Design review of the part built by this model. Coordinates are the model's own, in mm. A direction names the side the tool comes from. Round coordinates to 2 decimals unless told otherwise and drop trailing zeros. Loops run counter-clockwise (first coordinate to the right, second up) from the corner with the lowest first, then second, coordinate; pieces in that order, holes last. Notation, with made-up numbers: (29.5, 34.5) -> (68.5, 34.5) arc R24 cw to (68.5, 55.5) -> close; hole circle Ø4 at (-20, 63). An arc over 180 degrees is marked (long way). Answer as CSV lines item,"result". Start each with the question number.
(1) Take a section at B-B, the plane z = 10. Write out the cut boundary in (x, y), and give its area (3 significant figures).
(2) For P1, Ø4, axis at x = 43, y = 15.5, coming from the -Z side; P2, Ø12, axis at y = 11.5, z = 23.5, coming from the -X side; P3, Ø5, axis at y = 8.5, z = 10.5, coming from the -X side, all flat-tipped, find the tip position at first contact; note any pin that passes through.
(3) Take a section at D-D, the plane z = -10. Write out the cut boundary in (x, y).
(4) Take a section at C-C, the plane y = 28. Write out the cut boundary in (x, z).
(5) Take a section at A-A, the plane x = 35. Write out the cut boundary in (y, z).
(6) Machinability: for faces 1 (the face through (-39.643, 17.283, -13.252)), 2 (the face through (-38, 34, 11)), which of the approach directions +Z, -Z, +X, -X, +Y, -Y give a long, thin tool a straight path to every point of the face, cutting with its end or side? Answer none if there is none.
(7) To check wall thickness, follow line 1 (X direction, y = 13, z = 10); line 2 (Z direction, x = 35, y = 12); line 3 (X direction, y = 24.5, z = -10). State the ranges of each line that lie inside material, in increasing order. Write a range as from..to.
(8) Draft analysis for pull direction X (two halves, no side actions). For faces 3 (the face through (-11.581, 1.875, -3.021)), 4 (the face through (30, 17, 40)), 5 (the face through (-40, 16, 12)), state which applies: +X half, -X half, draft (parallel to the pull), parting line (faces both ways), or undercut.
from build123d import *
from OCP.BRepFilletAPI import BRepFilletAPI_MakeChamfer

# Parameters (mm, degrees)
BOSS_EXTRUDE1_DEPTH     = 35
CUT_EXTRUDE3_DEPTH      = 84.964278119
CUT_EXTRUDE3_DEPTH_BACK = 84.964278119
SKETCH2_R               = 12.5
SKETCH2_R_2             = 15
CHAMFER1_SIZE           = 3
CHAMFER2_SIZE           = 2
CHAMFER3_SIZE           = 5
CHAMFER3_SIZE2          = 2.886751346
FILLET1_R               = 5


with BuildPart() as part:
    # Sketch1 → Boss-Extrude1 (new body)
    with BuildSketch(Plane(origin=(0, 0, 0), x_dir=(1, 0, 0), z_dir=(0, 1, 0))):
        with BuildLine():
            Line((-40, -16.905989232), (0, -40))
            Line((0, -40), (65, -40))
            Line((65, -40), (65, 20))
            Line((65, 20), (-4.844355629, 20))
            ThreePointArc((-4.844355629, 20), (-38.631222116, 27.900831925), (-40, -6.770509831))
            Line((-40, -6.770509831), (-40, -16.905989232))
        make_face()
    extrude(amount=BOSS_EXTRUDE1_DEPTH)

    # Sketch2 → Cut-Extrude3 (cut, two sides: drawn at the far end of the back side and taken through both)
    with BuildSketch(Plane(origin=(0, 0, 0), x_dir=(1, 0, 0), z_dir=(0, 1, 0)).offset(-CUT_EXTRUDE3_DEPTH_BACK)):
        with Locations(Location((35, -10, 0), (0, 0, 270))):
            Circle(SKETCH2_R)
        with Locations(Location((-25, 10, 0), (0, 0, 270))):
            Circle(SKETCH2_R_2)
    extrude(amount=CUT_EXTRUDE3_DEPTH + CUT_EXTRUDE3_DEPTH_BACK, mode=Mode.SUBTRACT)

    # Chamfer1
    chamfer1_edges = [part.edges().sort_by_distance(p)[0] for p in [
        (-20, 35, 28.452994616),
        (-40, 35, 11.838249532),
        (-38.631222116, 35, -27.900831925),
    ]]
    chamfer(chamfer1_edges, length=CHAMFER1_SIZE)

    # Chamfer2
    chamfer2_edges = [part.edges().sort_by_distance(p)[0] for p in [
        (-25, 0, -25),
        (-25, 35, -25),
    ]]
    chamfer(chamfer2_edges, length=CHAMFER2_SIZE)

    # Chamfer3: one chamfer whose edges measure the first distance from different faces: ONE call of the kernel's chamfer builder (chamfer() names one face for all edges)
    chamfer3_edges_1 = [part.edges().sort_by_distance(p)[0] for p in [
        (35, 0, -2.5),
    ]]
    chamfer3_side_1 = [part.faces().sort_by_distance(p)[0] for p in [
        (35, 17.5, -2.5),
    ]]
    chamfer3_edges_2 = [part.edges().sort_by_distance(p)[0] for p in [
        (35, 35, -2.5),
    ]]
    chamfer3_side_2 = [part.faces().sort_by_distance(p)[0] for p in [
        (20.131502665, 35, 9.160583392),
    ]]
    chamfer3 = BRepFilletAPI_MakeChamfer(part.part.solid().wrapped)
    for e in chamfer3_edges_1:
        chamfer3.Add(CHAMFER3_SIZE, CHAMFER3_SIZE2, e.wrapped, chamfer3_side_1[0].wrapped)  # the first distance lies on this face
    for e in chamfer3_edges_2:
        chamfer3.Add(CHAMFER3_SIZE, CHAMFER3_SIZE2, e.wrapped, chamfer3_side_2[0].wrapped)  # the first distance lies on this face
    add(Compound.cast(chamfer3.Shape()), mode=Mode.REPLACE)

    # Fillet1
    fillet1_edges = [part.edges().sort_by_distance(p)[0] for p in [
        (65, 17.5, 40),
        (65, 17.5, -20),
        (-4.844355629, 16, -20),
    ]]
    fillet(fillet1_edges, radius=FILLET1_R)


solid = part.part
The answers:
1,outline,"(-40, 0) -> (19.61, 0) -> (22.5, 5) -> (22.5, 32.11) -> (17.5, 35) -> (-37, 35) -> (-40, 32) -> close; (47.5, 5) -> (50.39, 0) -> (65, 0) -> (65, 35) -> (52.5, 35) -> (47.5, 32.11) -> close"
1,area,"2,770 mm²"
2,P1,"z = -20"
2,P2,"x = -38.97"
2,P3,"x = -40"
3,outline,"(-47.5, 0) -> (-42, 0) -> (-40, 2) -> (-40, 33) -> (-42, 35) -> (-44.5, 35) -> (-47.5, 32) -> close; (-10, 2) -> (-8, 0) -> (65, 0) -> (65, 35) -> (-8, 35) -> (-10, 33) -> close"
4,outline,"(-40, 6.77) arc R22.5 ccw (long way) to (-6.14, -22.27) arc R5 cw to (-1.95, -20) -> (60, -20) arc R5 ccw to (65, -15) -> (65, 35) arc R5 ccw to (60, 40) -> (0, 40) -> (-40, 16.91) -> close; hole circle Ø30 at (-25, -10); hole circle Ø25 at (35, 10)"
5,outline,"(0, -20) -> (35, -20) -> (35, -7.5) -> (32.11, -2.5) -> (5, -2.5) -> (0, -5.39) -> close; (0, 25.39) -> (5, 22.5) -> (32.11, 22.5) -> (35, 27.5) -> (35, 40) -> (0, 40) -> close"
6,face 1,"+Y, -Y"
6,face 2,"+Z, -X, +Y"
7,line 1,"-40..22.5, 47.5..65"
7,line 2,"-20..-2.5, 22.5..40"
7,line 3,"-47.5..-40, -10..65"
8,face 3,"undercut"
8,face 4,"draft"
8,face 5,"-X half"
